The listing builds one solid part. Answer for the finished solid, in the listing's coordinates (mm). Face numbers are marked on the shaded views. Give positions to 0.01 mm unless a question says otherwise; leave off trailing zeros. Loops run counter-clockwise (first coordinate to the right, second up) from the corner with the lowest first, then second, coordinate; pieces in that order, holes last.
Item 1: Section C-C, the plane x = 787 is taken. Give the vertices of the cut face in (y, z).
Item 2: The mould has two halves that part along Z. Classify the marked faces 1, 2 and 3: pulls with the +Z half, pulls with the -Z half, needs draft (parallel to the pull), parting line crosses it, or undercut.
Item 3: Section B-B, the plane z = -1.5 is taken. Give the vertices of the cut face in (x, y), and give its area (4 significant figures).
Item 4: Section A-A, the plane y = -14.5 is taken. Give the vertices of the cut face in (x, z).
Item 5: Consider line 1 along Y through (x, z) = (339, 14.5); line 2 along Z through (x, y) = (1022, -13.5); line 3 along X through (y, z) = (6, 31.5). Determine where each line is inside the solid, lowest interval first.
from build123d import *

# Parameters (mm, degrees)
SKETCH_2_W          = 70
SKETCH_2_H          = 75
SKETCH_2_W_2        = 60
SKETCH_2_H_2        = 65
EXTRUDE_1_DEPTH     = 1400
SKETCH_3_OUTSIDE_W  = 1682.75
SKETCH_3_OUTSIDE_H  = 357.75
CUT_EXTRUDE_1_DEPTH = 71


with BuildPart() as part:
    # Эскиз2 → Вытянуть-Тонкостенный1 (new body)
    with BuildSketch(Plane(origin=(0, 0, 0), x_dir=(0, 0, -1), z_dir=(1, 0, 0))):
        Rectangle(SKETCH_2_W, SKETCH_2_H)
        Rectangle(SKETCH_2_W_2, SKETCH_2_H_2, mode=Mode.SUBTRACT)
    extrude(amount=EXTRUDE_1_DEPTH)

    # Эскиз3 outside → Вырез-Вытянуть1 (cut, through all)
    with BuildSketch(Plane(origin=(0, 0, -35), x_dir=(-1, 0, 0), z_dir=(0, 0, -1))):
        with Locations((-700, 0)):
            Rectangle(SKETCH_3_OUTSIDE_W, SKETCH_3_OUTSIDE_H)
        Polygon((-1400, -37.5), (-1325, 37.5), (-75, 37.5), (0, -37.5), align=None, mode=Mode.SUBTRACT)
    extrude(amount=-CUT_EXTRUDE_1_DEPTH, mode=Mode.SUBTRACT)


solid = part.part
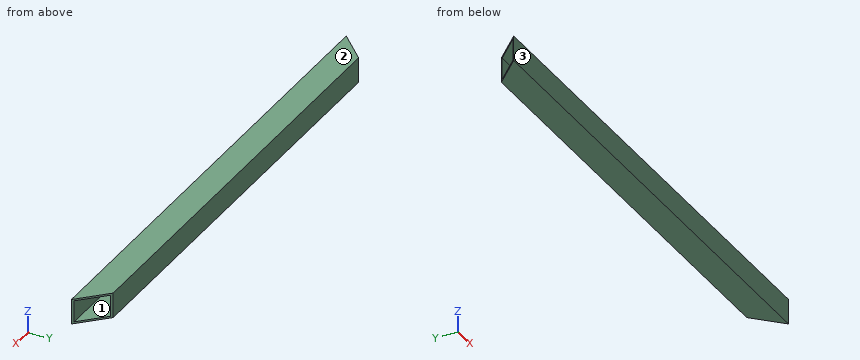
Worked answers:
1. outline: (-37.5, -35) - (37.5, -35) - (37.5, 35) - (-37.5, 35) - close; hole (-32.5, -30) - (32.5, -30) - (32.5, 30) - (-32.5, 30) - close
2. face 1: undercut
2. face 2: pulls with the +Z half
2. face 3: needs draft
3. outline: (0, -37.5) - (1400, -37.5) - (1395, -32.5) - (5, -32.5) - close; (70, 32.5) - (1330, 32.5) - (1325, 37.5) - (75, 37.5) - close
3. area: 13,250 mm2
4. outline: (23, -35) - (1377, -35) - (1377, -30) - (23, -30) - close; (23, 30) - (1377, 30) - (1377, 35) - (23, 35) - close
5. line 1: y = -37.5 to -32.5, 32.5 to 37.5
5. line 2: z = -35 to -30, 30 to 35
5. line 3: x = 43.5 to 1356.5
